```python
from build123d import *

# Parameters (mm, degrees)
CROQUIS1_R                 = 5
SALIENTE_EXTRUIR1_DEPTH    = 20
CORTAR_EXTRUIR1_DEPTH      = 7
CORTAR_EXTRUIR2_DEPTH      = 22.615966321
CORTAR_EXTRUIR2_DEPTH_BACK = 22.615966321
CROQUIS3_R                 = 1.5
CROQUIS4_R                 = 3.175
CORTAR_EXTRUIR3_DEPTH      = 13
REDONDEO1_R                = 1


with BuildPart() as part:
    # Croquis1 → Saliente-Extruir1 (new body)
    with BuildSketch(Plane(origin=(0, 0, 0), x_dir=(1, 0, 0), z_dir=(0, 1, 0))):
        with Locations(Location((0, 0, 0), (0, 0, 270))):
            Circle(CROQUIS1_R)
    extrude(amount=SALIENTE_EXTRUIR1_DEPTH)

    # Croquis2 → Cortar-Extruir1 (cut)
    with BuildSketch(Plane(origin=(0, 20, 0), x_dir=(1, 0, 0), z_dir=(0, 1, 0))):
        with BuildLine():
            Line((2.184605227, 1.5), (0, 1.5))
            Line((0, 1.5), (-2.184605227, 1.5))
            ThreePointArc((-2.184605227, 1.5), (-2.65, 0), (-2.184605227, -1.5))
            Line((-2.184605227, -1.5), (0, -1.5))
            Line((0, -1.5), (2.184605227, -1.5))
            ThreePointArc((2.184605227, -1.5), (2.530978452, -0.785269427), (2.65, 0))
            ThreePointArc((2.65, 0), (2.530978452, 0.785269427), (2.184605227, 1.5))
        make_face()
    extrude(amount=-CORTAR_EXTRUIR1_DEPTH, mode=Mode.SUBTRACT)

    # Croquis3 → Cortar-Extruir2 (cut, two sides: drawn at the far end of the back side and taken through both)
    with BuildSketch(Plane.XY.offset(-1.5).offset(-CORTAR_EXTRUIR2_DEPTH_BACK)):
        with Locations(Location((0, 16.5, 0), (0, 0, 90))):
            Circle(CROQUIS3_R)
    extrude(amount=CORTAR_EXTRUIR2_DEPTH + CORTAR_EXTRUIR2_DEPTH_BACK, mode=Mode.SUBTRACT)

    # Croquis4 → Cortar-Extruir3 (cut)
    with BuildSketch(Plane.XZ):
        with Locations(Location((0, 0, 0), (0, 0, 270))):
            Circle(CROQUIS4_R)
    extrude(amount=-CORTAR_EXTRUIR3_DEPTH, mode=Mode.SUBTRACT)

    # Redondeo1
    redondeo1_edges = [part.edges().sort_by_distance(p)[0] for p in [
        (0, 0, -5),
        (0, 20, -5),
    ]]
    fillet(redondeo1_edges, radius=REDONDEO1_R)


solid = part.part
```
The listing builds one solid part. Answer for the finished solid, in the listing's coordinates (mm). A direction names the side the tool comes from. Coordinates: 2 decimals unless noted, no trailing zeros. Write each loop counter-clockwise with the first axis right and the second up, starting at its lowest first coordinate (ties: lowest second). Pieces come first, ordered by that corner, then holes. Notation, with made-up numbers: (-33, 3) - (7, 3) arc R31 cw to (7, 27) - close; hole circle Ø8 at (-36, 40). An arc over 180 degrees is marked (long way). Return JSON: item names as keys, results as strings. Group by question number.
Q1. Which of the six approach directions +Z, -Z, +X, -X, +Y, -Y give full straight-line access (tool end or side, diameter ignored) to faces 4 (the flat face through (2, 0, -3)), 5 (the cylindrical face through (-1.93, 6.41, 2.52)), 6 (the flat face through (-1, 15, 1.5))?
Q2. For a pull along Y with two mould halves and no side action, classify faces 1 (the cylindrical face through (-2.65, 16.55, -0.02)), 2 (the cylindrical face through (0, 18, 3)), 3 (the flat face through (0, 13, -2)) as +Y half, -Y half, draft (parallel to the pull), parting line (faces both ways), or undercut.
Q3. The part is cut by section B-B on y = 2.75. Write down the section's boundary in (x, z) (3 decimals), and give its area (3 significant figures).
Q4. The part is cut by section A-A on x = 0. Write down the section's boundary in (y, z) (3 decimals), and give its area (3 significant figures).
Q5. The part is cut by section C-C on y = 16.5. Write down the section's boundary in (x, z), and give its area (3 significant figures).
Q6. Find the intervals of material crossed by line 1 along X through (y, z) = (3, 0) (3 decimals); line 2 along Y through (x, z) = (0, 3.8); line 3 along Z through (x, y) = (1, 13.5), in increasing order. Write a range as [from, to].
Q7. Flat-ended cylindrical pins translate along their axes: pin 1 Ø5 at (x, z) = (0, 0) entering from -Y; pin 2 Ø1.3 at (x, y) = (0, 16.5) entering from +Z; pin 3 Ø4 at (y, z) = (5, -3) entering from -X; pin 4 Ø1.5 at (y, z) = (4, -3) entering from +X. Find the tip coordinate at first contact, or state that the pin passes through.
Evaluation:
{
 "1": {"face 4": "+Z, -Z, +X, -X, -Y", "face 5": "-Y", "face 6": "+Y, -Y"},
 "2": {"face 1": "draft", "face 2": "undercut", "face 3": "-Y half"},
 "3": {"outline": "circle Ø10 at (0, 0); hole circle Ø6.35 at (0, 0)", "area": "46.9 mm2"},
 "4": {"outline": "(0, -4) arc R1 ccw to (1, -5) - (15, -5) - (15, -1.5) - (13, -1.5) - (13, -3.175) - (0, -3.175) - close; (0, 3.175) - (13, 3.175) - (13, 1.5) - (15, 1.5) - (15, 5) - (1, 5) arc R1 ccw to (0, 4) - close; (18, -5) - (19, -5) arc R1 ccw to (20, -4) - (20, -1.5) - (18, -1.5) - close; (18, 1.5) - (20, 1.5) - (20, 4) arc R1 ccw to (19, 5) - (18, 5) - close", "area": "74.6 mm2"},
 "5": {"outline": "(-2.18, -1.5) arc R2.65 cw to (-2.18, 1.5) - (-1.5, 1.5) - (-1.5, 4.77) arc R5 ccw to (-1.5, -4.77) - (-1.5, -1.5) - close; (1.5, -4.77) arc R5 ccw to (1.5, 4.77) - (1.5, 1.5) - (2.18, 1.5) arc R2.65 cw to (2.18, -1.5) - (1.5, -1.5) - close", "area": "43.0 mm2"},
 "6": {"line 1": "x = [-5, -3.175], [3.175, 5]", "line 2": "y = [0, 15], [18, 20]", "line 3": "z = [-4.9, -1.5], [1.5, 4.9]"},
 "7": {"pin 1": "stops at y = 13", "pin 2": "passes through", "pin 3": "stops at x = -4.9", "pin 4": "stops at x = 4.47"}
}
